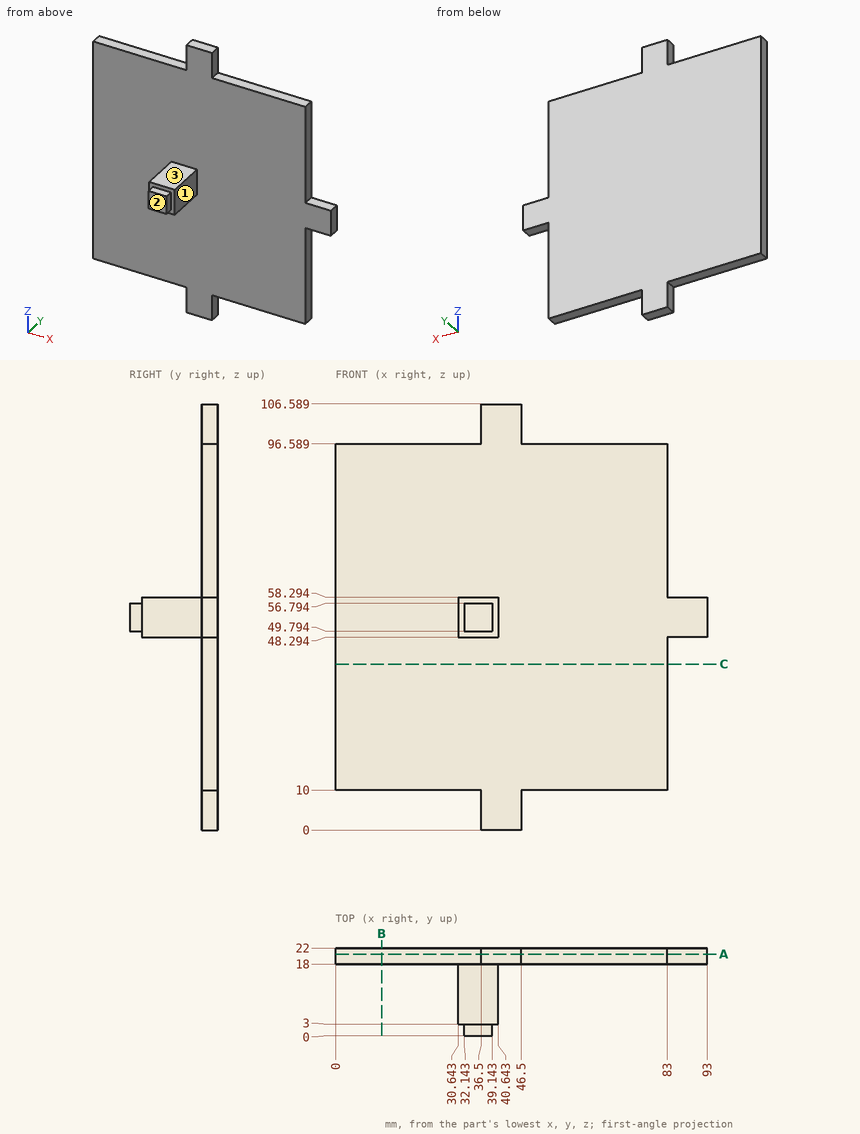
Here's the drawing with two shaded views (mm, measured from the low corner). I have some questions. A direction names the side the tool comes from. Coordinates: 2 decimals unless noted, no trailing zeros. Write each loop counter-clockwise with the first axis right and the second up, starting at its lowest first coordinate (ties: lowest second). Pieces come first, ordered by that corner, then holes.
Item 1: I want a section at B-B on x = 11.5. Write out the boundary of the cut face in (y, z).
Item 2: Will these pins go through, and if not, where does the flat tip stop? pin 1 (3 mm diameter, centred on x = 40.5, y = 10.5, fed in from +Z); pin 2 (6 mm diameter, centred on x = 57.5, z = 15, fed in from -Y); pin 3 (2 mm diameter, centred on y = 19.5, z = 78, fed in from +X).
Item 3: On a 3-axis mill with a long thin cutter (end or side, diameter ignored), from which of +Z, -Z, +X, -X, +Y, -Y can I reach the whole of each face in a straight line? I mean the marked faces 1, 2 and 3. Say none if no direction works.
Item 4: If I drill on line 1 (Y direction, x = 67.5, z = 45.5); line 2 (Z direction, x = 53, y = 20.5); line 3 (Z direction, x = 31, y = 13) (1 decimal), over which ranges is the centre line in solid material (lowest first)?
Item 5: I want a section at A-A on y = 20.5. Write out the boundary of the cut face in (x, z) (1 decimal), and give its area (3 significant figures).
Item 6: I want a section at C-C on z = 41.5. Write out the boundary of the cut face in (x, y).
Findings below:
1. outline: (18, 10) - (22, 10) - (22, 96.59) - (18, 96.59) - close
2. pin 1: stops at z = 58.29
2. pin 2: stops at y = 18
2. pin 3: stops at x = 83
3. face 1: +Z, -Z, +X, -Y
3. face 2: +Z, -Z, +X, -X, -Y
3. face 3: +Z, +X, -X, -Y
4. line 1: y = 18 to 22
4. line 2: z = 10 to 96.59
4. line 3: z = 48.3 to 58.3
5. outline: (0, 10) - (36.5, 10) - (36.5, 0) - (46.5, 0) - (46.5, 10) - (83, 10) - (83, 48.3) - (93, 48.3) - (93, 58.3) - (83, 58.3) - (83, 96.6) - (46.5, 96.6) - (46.5, 106.6) - (36.5, 106.6) - (36.5, 96.6) - (0, 96.6) - close
5. area: 7,490 mm2
6. outline: (0, 18) - (83, 18) - (83, 22) - (0, 22) - close
